Autodesk Inventor part; units mm, degrees
ref_plane "YZ Plane" through (0, 0, 0) normal (1, 0, 0) x (0, 1, 0)
ref_plane "XZ Plane" through (0, 0, 0) normal (0, 1, 0) x (-1, 0, 0)
ref_plane "XY Plane" through (0, 0, 0) normal (0, 0, 1) x (1, 0, 0)
sketch "Эскиз1" plane through (0, 0, 0) normal (0, 1, 0) x (-1, 0, 0)
  circle A0 centre (0, 0) radius 15
  circle A1 centre (0, 0) radius 12.75
  dimension "d0" = 30
  dimension "d1" = 25.5
extrude "Выдавливание1" add sketch "Эскиз1" along normal blind 50
sketch "Эскиз2" plane through (0, 0, 0) normal (0, -1, 0) x (1, 0, 0)
  circle A0 centre (0, 0) radius 15
extrude "Выдавливание2" add sketch "Эскиз2" against normal blind 42
sketch "Эскиз3" plane through (0, 0, 0) normal (0, -1, 0) x (1, 0, 0)
  circle A0 centre (-5.5, -5) radius 1.25
  circle A1 centre (5.5, -5) radius 1.25
  circle A2 centre (-5.5, 5) radius 1.25
  circle A3 centre (5.5, 5) radius 1.25
  line L0 (5.5, 5) -> (-5.5, 5)
  line L1 (-5.5, 5) -> (-5.5, -5)
  line L2 (-5.5, -5) -> (5.5, -5)
  line L3 (5.5, -5) -> (5.5, 5)
  line L4 (5.5, -5) -> (-5.5, 5) construction
  point P0 (0, 0)
  point P1 (0, 0)
  dimension "d6" = 2.5
  dimension "d7" = 2.5
  dimension "d8" = 2.5
  dimension "d9" = 2.5
extrude "Выдавливание3" cut sketch "Эскиз3" against normal blind 15 contours L2 L1 A0 | A0 L1 L2 | L2 L3 A1 | A1 L3 L2 | L1 L0 A2 | A2 L0 L1 | L3 L0 A3 | A3 L0 L3
sketch "Эскиз4" plane through (0, 42, 0) normal (0, 1, 0) x (1, 0, 0)
  circle A0 centre (0, 0) radius 2.65
  dimension "d12" = 5.3
extrude "Выдавливание4" cut sketch "Эскиз4" against normal through all
sketch "Эскиз5" plane through (0, 0, 0) normal (0, 0, 1) x (1, 0, 0)
  line L0 (-4, 37) -> (4, 37)
  line L1 (4, 37) -> (4, 33)
  line L2 (4, 33) -> (-4, 33)
  line L3 (-4, 33) -> (-4, 37)
  line L4 (-4, 37) -> (4, 33) construction
  line L5 (4, 37) -> (-4, 33) construction
  point P0 (0, 0)
  point P1 (0, 35)
  dimension "d15" = 4
  dimension "d16" = 8
extrude "Выдавливание5" cut sketch "Эскиз5" along normal through all both and the other way through all
chamfer "Фаска1" distance 2 angle 45 8 edges at (0, 33, 15) (0, 33, -15) (-4, 35, 14.4568) (-4, 35, -14.4568) (0, 37, 15) (0, 37, -15) (4, 35, 14.4568) (4, 35, -14.4568)
properties part number "магнит_стойка"
Input: part model. Units: mm. Frame: model coordinates. A direction names the side the tool comes from. Round coordinates to 2 decimals unless told otherwise and drop trailing zeros. Order: outer loops, then holes, each group sorted by start corner. A loop starts at its lowest first (then second) coordinate and runs counter-clockwise, first axis right, second up. Notation, with made-up numbers: (82, 3) - (117, 3) arc R20 cw to (117, 37) - close; hole circle Ø7 at (-40, 44). An arc over 180 degrees is marked (long way). Answer in a Markdown table with one row per item.
Item 1: Reachability of faces 1 (the conical face through (0, 38, -14)), 2 (the cylindrical face through (5.23, 7.4, -6.22)), 3 (the conical face through (0, 32, 14)) from +Z, -Z, +X, -X, +Y, -Y: full face, straight path, thin tool, end or side. Return the list, or none.
Model answer:
| item | result |
|---|---|
| face 1 | -Z |
| face 2 | -Y |
| face 3 | +Z |
Item 2: Section query C-C (y = 13). Return the cut outline in (x, z).
Model answer:
| item | result |
|---|---|
| outline | circle Ø30 at (0, 0); hole circle Ø2.5 at (-5.5, -5); hole circle Ø2.5 at (-5.5, 5); hole circle Ø5.3 at (0, 0); hole circle Ø2.5 at (5.5, -5); hole circle Ø2.5 at (5.5, 5) |
Item 3: Section query A-A (x = 0). Return the cut outline in (y, z), then the cut area to 3 significant figures.
Model answer:
| item | result |
|---|---|
| outline | (0, -15) - (31, -15) - (33, -13) - (33, -2.65) - (0, -2.65) - close; (0, 2.65) - (33, 2.65) - (33, 13) - (31, 15) - (0, 15) - close; (37, -13) - (39, -15) - (50, -15) - (50, -12.75) - (42, -12.75) - (42, -2.65) - (37, -2.65) - close; (37, 2.65) - (42, 2.65) - (42, 12.75) - (50, 12.75) - (50, 15) - (39, 15) - (37, 13) - close |
| area | 967 mm² |
Item 4: Pin query (flat end, axial travel): pin 1 (2 mm diameter, centred on x = -5.5, z = 5, fed in from -Y); pin 2 (2 mm diameter, centred on x = -6, z = -4.5, fed in from -Y); pin 3 (10 mm diameter, centred on x = -11.5, y = 41.5, fed in from -Z); pin 4 (4 mm diameter, centred on x = 5.5, z = -5, fed in from +Y). Return the tip coordinate at first contact, or that it passes through.
Model answer:
| item | result |
|---|---|
| pin 1 | stops at y = 15 |
| pin 2 | stops at y = 0 |
| pin 3 | stops at z = -13.52 |
| pin 4 | stops at y = 42 |
Item 5: Section query B-B (z = 0). Return the cut outline in (x, y).
Model answer:
| item | result |
|---|---|
| outline | (-15, 0) - (-2.65, 0) - (-2.65, 33) - (-4, 33) - (-4, 37) - (-2.65, 37) - (-2.65, 42) - (-12.75, 42) - (-12.75, 50) - (-15, 50) - close; (2.65, 0) - (15, 0) - (15, 50) - (12.75, 50) - (12.75, 42) - (2.65, 42) - (2.65, 37) - (4, 37) - (4, 33) - (2.65, 33) - close |
Item 6: Line query: line 1 (Z direction, x = -5.5, y = 5.5); line 2 (Y direction, x = -1, z = -4); line 3 (X direction, y = 9, z = 5). Output: solid intervals per line, ascending.
Model answer:
| item | result |
|---|---|
| line 1 | z = -13.96 to -6.25, -3.75 to 3.75, 6.25 to 13.96 |
| line 2 | y = 0 to 33, 37 to 42 |
| line 3 | x = -14.14 to -6.75, -4.25 to 4.25, 6.75 to 14.14 |
Item 7: Mould query, pull axis X, two halves, no side actions, for faces 4 (the flat face through (7, 50, -11)), 5 (the flat face through (-6, 15, -5)). Classes: released by +X, released by -X, zero draft, split by the parting line, or undercut.
Model answer:
| item | result |
|---|---|
| face 4 | zero draft |
| face 5 | undercut |
Item 8: Section query D-D (z = 5). Return the cut outline in (x, y), then the cut area to 3 significant figures.
Model answer:
| item | result |
|---|---|
| outline | (-14.14, 0) - (-6.75, 0) - (-6.75, 15) - (-4.25, 15) - (-4.25, 0) - (4.25, 0) - (4.25, 15) - (6.75, 15) - (6.75, 0) - (14.14, 0) - (14.14, 50) - (11.73, 50) - (11.73, 42) - (-11.73, 42) - (-11.73, 50) - (-14.14, 50) - close; hole (-4, 33) - (4, 33) - (4, 37) - (-4, 37) - close |
| area | 1,120 mm² |
